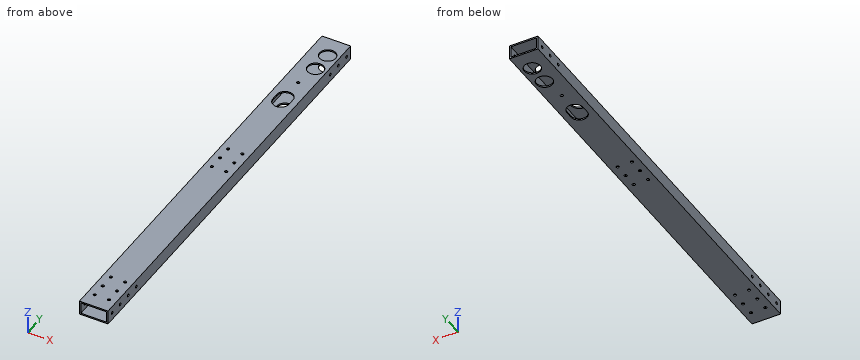
```python
from build123d import *

# Parameters (mm, degrees)
F0_W     = 50.8
F0_H     = 25.4
F0_W_2   = 45.72
F0_H_2   = 20.32
F1_DEPTH = 787.4
F3_R     = 14.2875
F3_R_2   = 2.4892
F3_R_3   = 2.5527
F4_DEPTH = 25.4
F2_R     = 2.5527
F5_DEPTH = 50.801
F6_DEPTH = 25.4


# Not quite as in the source:
# - a feature names something its author has since deleted; it is built from what else it names


with BuildPart() as f1:
    # F0 (on Front) → F1 (new body)
    with BuildSketch(Plane.XZ):
        with Locations((25.4, 12.7)):
            Rectangle(F0_W, F0_H)
        with Locations((25.4, 12.7)):
            Rectangle(F0_W_2, F0_H_2, mode=Mode.SUBTRACT)
    extrude(amount=F1_DEPTH)

    # F3 (on face) → F4 (cut)
    with BuildSketch(Plane.XY.offset(25.4)):
        with Locations((31.75, -63.5)):
            Circle(F3_R)
        with BuildLine():
            ThreePointArc((38.1988341754, -193.04), (39.3103558461, -189.9510821033), (39.6875, -186.69))
            ThreePointArc((39.6875, -186.69), (25.4, -172.4025), (11.1125, -186.69))
            ThreePointArc((11.1125, -186.69), (11.4896441539, -189.9510821033), (12.6011658246, -193.04))
            ThreePointArc((12.6011658246, -193.04), (25.4, -185.1025), (38.1988341754, -193.04))
        make_face()
        with BuildLine():
            Line((39.6875, -199.39), (39.6875, -186.69))
            ThreePointArc((39.6875, -186.69), (39.3103558461, -189.9510821033), (38.1988341754, -193.04))
            ThreePointArc((38.1988341754, -193.04), (39.3103558461, -196.1289178967), (39.6875, -199.39))
        make_face()
        with BuildLine():
            ThreePointArc((12.6011658246, -193.04), (11.4896441539, -189.9510821033), (11.1125, -186.69))
            Line((11.1125, -186.69), (11.1125, -199.39))
            ThreePointArc((11.1125, -199.39), (11.4896441539, -196.1289178967), (12.6011658246, -193.04))
        make_face()
        with BuildLine():
            ThreePointArc((39.6875, -199.39), (39.3103558461, -196.1289178967), (38.1988341754, -193.04))
            ThreePointArc((38.1988341754, -193.04), (25.4, -200.9775), (12.6011658246, -193.04))
            ThreePointArc((12.6011658246, -193.04), (11.4896441539, -196.1289178967), (11.1125, -199.39))
            ThreePointArc((11.1125, -199.39), (25.4, -213.6775), (39.6875, -199.39))
        make_face()
        with BuildLine():
            ThreePointArc((12.6011658246, -193.04), (25.4, -200.9775), (38.1988341754, -193.04))
            ThreePointArc((38.1988341754, -193.04), (25.4, -185.1025), (12.6011658246, -193.04))
        make_face()
        with Locations((12.7, -736.6)):
            Circle(F3_R_2)
        with Locations((12.7, -711.2)):
            Circle(F3_R_2)
        with Locations((38.1, -736.6)):
            Circle(F3_R_2)
        with Locations((38.1, -711.2)):
            Circle(F3_R_2)
        with Locations((12.7, -342.9)):
            Circle(F3_R_3)
        with Locations((12.7, -368.3)):
            Circle(F3_R_3)
        with Locations((12.7, -393.7)):
            Circle(F3_R_3)
        with Locations((38.1, -342.9)):
            Circle(F3_R_3)
        with Locations((38.1, -368.3)):
            Circle(F3_R_3)
        with Locations((38.1, -393.7)):
            Circle(F3_R_3)
        with Locations((25.4, -145.034)):
            Circle(F3_R_2)
        with Locations((38.1, -762)):
            Circle(F3_R_2)
        with Locations((12.7, -762)):
            Circle(F3_R_2)
        with Locations((31.75, -101.6)):
            Circle(F3_R)
    extrude(amount=-F4_DEPTH, mode=Mode.SUBTRACT)

    # F2 (on face) → F5 (cut, through all)
    with BuildSketch(Plane.YZ.offset(50.8)):
        with Locations((-12.7, 12.7)):
            Circle(F2_R)
        with Locations((-38.1, 12.7)):
            Circle(F2_R)
        with Locations((-63.5, 12.7)):
            Circle(F2_R)
        with Locations((-88.9, 12.7)):
            Circle(F2_R)
        with Locations((-774.7, 12.7)):
            Circle(F2_R)
        with Locations((-749.3, 12.7)):
            Circle(F2_R)
        with Locations((-723.9, 12.7)):
            Circle(F2_R)
        with Locations((-698.5, 12.7)):
            Circle(F2_R)
    extrude(amount=-F5_DEPTH, mode=Mode.SUBTRACT)

    # F0 (on Front) → F6 (cut)
    with BuildSketch(Plane.XZ):
        with Locations((25.4, 12.7)):
            Rectangle(F0_W, F0_H)
        with Locations((25.4, 12.7)):
            Rectangle(F0_W_2, F0_H_2, mode=Mode.SUBTRACT)
    extrude(amount=F6_DEPTH, mode=Mode.SUBTRACT)


solid = f1.part
```
CAD build for the part. Positions are in the model's coordinates, mm. Give positions to 0.01 mm unless a question says otherwise; leave off trailing zeros. Order: outer loops, then holes, each group sorted by start corner. A loop starts at its lowest first (then second) coordinate and runs counter-clockwise, first axis right, second up.
(1) Drill centre lines: L1, parallel to X at y = -736.6, z = 0.5; L2, parallel to X at y = -342.9, z = 1.4; L3, parallel to Z at x = 29, y = -372. Where is each one in solid material? Low to high.
(2) Flat gauge pin, fed straight in: pin 1 (8 mm diameter, centred on x = 12.7, y = -393.7, fed in from -Z). Where does the tip first touch, or does it go through?
(3) Saw through at A-A, the plane y = -281.5. Give the cut face in (x, z).
Results found:
1. L1: x = 0 to 10.21, 15.19 to 35.61, 40.59 to 50.8
1. L2: x = 0 to 10.15, 15.25 to 35.55, 40.65 to 50.8
1. L3: z = 0 to 2.54, 22.86 to 25.4
2. pin 1: stops at z = 0
3. outline: (0, 0) - (50.8, 0) - (50.8, 25.4) - (0, 25.4) - close; hole (2.54, 2.54) - (48.26, 2.54) - (48.26, 22.86) - (2.54, 22.86) - close
